from build123d import *

# Parameters (mm, degrees)
SKETCH1_R               = 4.5000037
BOSS_EXTRUDE1_DEPTH     = 3.75000012
BOSS_EXTRUDE2_START     = 1.750000056
SKETCH2_R               = 4.5000037
SKETCH2_R_2             = 3.499999998
SKETCH2_R_3             = 1.25000004
BOSS_EXTRUDE2_DEPTH     = 1.750000056
SKETCH4_R               = 2.75000466
SKETCH4_R_2             = 1.25000004
CUT_EXTRUDE1_DEPTH      = 0.875000028
SKETCH6_R               = 4.5000037
SKETCH6_R_2             = 3.5000057
CUT_EXTRUDE2_DEPTH      = 0.875000028
SKETCH10_R              = 0.62500002
SKETCH10_R_2            = 4.5000037
BOSS_EXTRUDE4_DEPTH     = 1.750000056
CHAMFER2_SIZE           = 1.00000054
CHAMFER2_SIZE2          = 0.577350581
ESQUISSE1_R             = 2.999994
ENL_V_MAT_EXTRU_1_DEPTH = 3.75000012


with BuildPart() as part:
    # Sketch1 → Boss-Extrude1 (new body)
    with BuildSketch(Plane.XY):
        with Locations((-10.24995918, 0)):
            Circle(SKETCH1_R)
        Polygon((-10.24995918, 2.999994), (-10.594624819, 2.728309468), (-10.996027349, 2.905743672), (-11.262299488, 2.55687975), (-11.695217312, 2.628914782), (-11.866365092, 2.224791874), (-12.303596391, 2.186901508), (-12.368865968, 1.752912142), (-12.782937891, 1.60747717), (-12.738228138, 1.170890494), (-13.103123023, 0.927049129), (-12.951243218, 0.515297489), (-13.244033377, 0.188371182), (-12.994526687, -0.172673551), (-13.196815038, -0.562142819), (-12.865358886, -0.849794878), (-12.964434908, -1.27733532), (-12.571855902, -1.473520467), (-12.561494285, -1.912268145), (-12.132459609, -2.004659346), (-12.01331141, -2.427046129), (-11.574778889, -2.409838105), (-11.354330629, -2.789323879), (-10.933854876, -2.663597874), (-10.625958129, -2.976338151), (-10.24995918, -2.749993992), (-9.873960231, -2.976338151), (-9.566063484, -2.663597874), (-9.145587731, -2.789323879), (-8.925139471, -2.409838105), (-8.48660695, -2.427046129), (-8.367458751, -2.004659346), (-7.938424075, -1.912268145), (-7.928062458, -1.473520467), (-7.535483452, -1.27733532), (-7.634559474, -0.849794878), (-7.303103322, -0.562142819), (-7.505391673, -0.172673551), (-7.255884983, 0.188371182), (-7.548675142, 0.515297489), (-7.396795337, 0.927049129), (-7.761690222, 1.170890494), (-7.716980469, 1.60747717), (-8.131052392, 1.752912142), (-8.196321969, 2.186901508), (-8.633553268, 2.224791874), (-8.804701048, 2.628914782), (-9.237618872, 2.55687975), (-9.503891011, 2.905743672), (-9.905293541, 2.728309468), align=None, mode=Mode.SUBTRACT)
    extrude(amount=-BOSS_EXTRUDE1_DEPTH)

    # Sketch2 → Boss-Extrude2 (add)
    # profile 1 of 2: a face of its own
    with BuildSketch(Plane.XY.offset(BOSS_EXTRUDE2_START)):
        with Locations((-10.24995918, 0)):
            Circle(SKETCH2_R)
        with Locations((-10.24995918, 0)):
            Circle(SKETCH2_R_2, mode=Mode.SUBTRACT)
    # profile 2 of 2: a face of its own
    with BuildSketch(Plane.XY.offset(BOSS_EXTRUDE2_START)):
        with Locations((-10.24995918, 0)):
            Circle(SKETCH2_R_2)
        with Locations((-10.24995918, 0)):
            Circle(SKETCH2_R_3, mode=Mode.SUBTRACT)
    extrude(amount=-BOSS_EXTRUDE2_DEPTH)

    # Sketch4 → Cut-Extrude1 (cut)
    with BuildSketch(Plane.XY.offset(1.750000056)):
        with Locations((-10.24995918, 0)):
            Circle(SKETCH4_R)
        with Locations((-10.24995918, 0)):
            Circle(SKETCH4_R_2, mode=Mode.SUBTRACT)
    extrude(amount=-CUT_EXTRUDE1_DEPTH, mode=Mode.SUBTRACT)

    # Sketch6 → Cut-Extrude2 (cut)
    with BuildSketch(Plane.XY.offset(1.750000056)):
        with Locations((-10.24995918, 0)):
            Circle(SKETCH6_R)
        with Locations((-10.24995918, 0)):
            Circle(SKETCH6_R_2, mode=Mode.SUBTRACT)
    extrude(amount=-CUT_EXTRUDE2_DEPTH, mode=Mode.SUBTRACT)

    # Sketch10 → Boss-Extrude4 (add)
    with BuildSketch(Plane.XY.offset(1.750000056)):
        with BuildLine():
            Line((-8.086927824, 17.701557226), (-6.029886341, 6.622035833))
            ThreePointArc((-6.029886341, 6.622035833), (-5.20161423, 5.04834495), (-3.627923347, 4.220072839))
            Line((-3.627923347, 4.220072839), (7.451598046, 2.163031356))
            ThreePointArc((7.451598046, 2.163031356), (9.25000182, 0), (7.451598046, -2.163031356))
            Line((7.451598046, -2.163031356), (-3.627923347, -4.220072839))
            ThreePointArc((-3.627923347, -4.220072839), (-5.20161423, -5.04834495), (-6.029886341, -6.622035833))
            Line((-6.029886341, -6.622035833), (-8.086927824, -17.701557226))
            ThreePointArc((-8.086927824, -17.701557226), (-10.24995918, -19.499961), (-12.412990536, -17.701557226))
            Line((-12.412990536, -17.701557226), (-14.470032019, -6.622035833))
            ThreePointArc((-14.470032019, -6.622035833), (-15.29830413, -5.04834495), (-16.871995013, -4.220072839))
            Line((-16.871995013, -4.220072839), (-27.951516406, -2.163031356))
            ThreePointArc((-27.951516406, -2.163031356), (-29.74992018, 0), (-27.951516406, 2.163031356))
            Line((-27.951516406, 2.163031356), (-16.871995013, 4.220072839))
            ThreePointArc((-16.871995013, 4.220072839), (-15.29830413, 5.04834495), (-14.470032019, 6.622035833))
            Line((-14.470032019, 6.622035833), (-12.412990536, 17.701557226))
            ThreePointArc((-12.412990536, 17.701557226), (-10.24995918, 19.499961), (-8.086927824, 17.701557226))
        make_face()
        with Locations((-10.24995918, 15.87496698)):
            Circle(SKETCH10_R, mode=Mode.SUBTRACT)
        with Locations((-10.24995918, 12.87497298)):
            Circle(SKETCH10_R, mode=Mode.SUBTRACT)
        with Locations((-10.24995918, 9.87497898)):
            Circle(SKETCH10_R, mode=Mode.SUBTRACT)
        with Locations((-10.24995918, 6.87498498)):
            Circle(SKETCH10_R, mode=Mode.SUBTRACT)
        with Locations((5.6250078, 0)):
            Circle(SKETCH10_R, mode=Mode.SUBTRACT)
        with Locations((2.6250138, 0)):
            Circle(SKETCH10_R, mode=Mode.SUBTRACT)
        with Locations((-0.3749802, 0)):
            Circle(SKETCH10_R, mode=Mode.SUBTRACT)
        with Locations((-3.3749742, 0)):
            Circle(SKETCH10_R, mode=Mode.SUBTRACT)
        with Locations((-10.24995918, -15.87496698)):
            Circle(SKETCH10_R, mode=Mode.SUBTRACT)
        with Locations((-10.24995918, -12.87497298)):
            Circle(SKETCH10_R, mode=Mode.SUBTRACT)
        with Locations((-10.24995918, -9.87497898)):
            Circle(SKETCH10_R, mode=Mode.SUBTRACT)
        with Locations((-10.24995918, -6.87498498)):
            Circle(SKETCH10_R, mode=Mode.SUBTRACT)
        with Locations((-26.12492616, 0)):
            Circle(SKETCH10_R, mode=Mode.SUBTRACT)
        with Locations((-23.12493216, 0)):
            Circle(SKETCH10_R, mode=Mode.SUBTRACT)
        with Locations((-20.12493816, 0)):
            Circle(SKETCH10_R, mode=Mode.SUBTRACT)
        with Locations((-17.12494416, 0)):
            Circle(SKETCH10_R, mode=Mode.SUBTRACT)
        with Locations((-10.24995918, 0)):
            Circle(SKETCH10_R_2, mode=Mode.SUBTRACT)
    extrude(amount=-BOSS_EXTRUDE4_DEPTH)

    # Chamfer2
    chamfer2_edges = [part.edges().sort_by_distance(p)[0] for p in [
        (-14.74996288, 0, 0),
    ]]
    chamfer2_side = [part.faces().sort_by_distance(p)[0] for p in [
        (-14.74996288, 0, -1.87500006),
    ]]
    chamfer(chamfer2_edges, length=CHAMFER2_SIZE, length2=CHAMFER2_SIZE2, reference=chamfer2_side[0])

    # Esquisse1 → Enlèv. mat.-Extru.1 (cut)
    with BuildSketch(Plane(origin=(0, 0, -3.75000012), x_dir=(-1, 0, 0), z_dir=(0, 0, -1))):
        with Locations((10.24995918, 0)):
            Circle(ESQUISSE1_R)
    extrude(amount=-ENL_V_MAT_EXTRU_1_DEPTH, mode=Mode.SUBTRACT)


solid = part.part
Model file for the job. Use its own axes, mm. A direction names the side the tool comes from. Coordinates: 2 decimals unless noted, no trailing zeros. Order: outer loops, then holes, each group sorted by start corner. A loop starts at its lowest first (then second) coordinate and runs counter-clockwise, first axis right, second up. Notation, with made-up numbers: (-37, -13) -> (8, -13) arc R31 ccw to (8, 18) -> close; hole circle Ø11 at (-22, 87). An arc over 180 degrees is marked (long way). Return JSON: item names as keys, results as strings. Group by question number.
Item 1: Saw through at C-C on y = 0. State how many separate pieces and enclosed holes the cut face has, then the cut area to 3 significant figures.
Item 2: Saw through at A-A on z = -2.05. Write the cut outline in (x, y).
Item 3: Pull direction Y, two halves, no side cores. Call faces 4 (the cylindrical face through (-10.746, 9.495, 0.887)), 5 (the flat face through (1.989, -3.177, 0.887)), 6 (the flat face through (-22.489, 3.177, 0.887)): pulls with the +Y half, pulls with the -Y half, needs draft (parallel to the pull), parting line crosses it, or undercut.
Item 4: Wall check: line 1 along Z through (x, y) = (-9, -9); line 2 along X through (y, z) = (14.5, 1.15); line 3 along Y through (x, z) = (-11.5, 1.15). Give the ranges that are in metal, low to high. Write a range as [from, to].
Item 5: Saw through at B-B on x = -23. Write the cut outline in (y, z).
Item 6: Tool access for faces 1 (the cylindrical face through (6.2, -0.24, 0.89)), 2 (the flat face through (-12, 0, 0)), 3 (the cylindrical face through (-12.277, 1.859, 1.319)): list every direction of +Z, -Z, +X, -X, +Y, -Y with a clear straight run to the whole face (end or side of a thin tool).
Item 7: Saw through at D-D on x = 4.5. Write the cut outline in (y, z).
Item 8: Flat gauge pins, fed straight in: P1, Ø1.7, axis at x = -10, y = -1, coming from the +Z side (3 decimals); P2, Ø3, axis at x = -10.25, y = 0, coming from the -Z side; P3, Ø3, axis at x = -8, z = -1, coming from the +Y side. Where does each tip first touch, or does it go through?
Values found:
{
 "1": {"separate pieces": "10", "enclosed holes": "0", "area": "53.8 mm2"},
 "2": {"outline": "circle Ø9 at (-10.25, 0); hole circle Ø6 at (-10.25, 0)"},
 "3": {"face 4": "undercut", "face 5": "pulls with the -Y half", "face 6": "pulls with the +Y half"},
 "4": {"line 1": "z = [0, 1.75]", "line 2": "x = [-13.01, -7.49]", "line 3": "y = [-19.11, -4.32], [-3.27, -2.45], [2.45, 3.27], [4.32, 19.11]"},
 "5": {"outline": "(-3.08, 0) -> (-0.61, 0) -> (-0.61, 1.75) -> (-3.08, 1.75) -> close; (0.61, 0) -> (3.08, 0) -> (3.08, 1.75) -> (0.61, 1.75) -> close"},
 "6": {"face 1": "+Z, -Z", "face 2": "-Z", "face 3": "+Z"},
 "7": {"outline": "(-2.71, 0) -> (2.71, 0) -> (2.71, 1.75) -> (-2.71, 1.75) -> close"},
 "8": {"P1": "stops at z = 0.875", "P2": "stops at z = 0", "P3": "stops at y = 19.19"}
}
